Job drawing, mm, ordinate dimensions from the low corner. One solid piece. Coordinates: 2 decimals unless noted, no trailing zeros. Order: outer loops, then holes, each group sorted by start corner. A loop starts at its lowest first (then second) coordinate and runs counter-clockwise, first axis right, second up. Notation, with made-up numbers: M 55,4 L 114,4 A21 cw 114,43 Z; hole C 64,4.5 d6. An arc over 180 degrees is marked long. Write item = value, one per line. Start each with the question number.
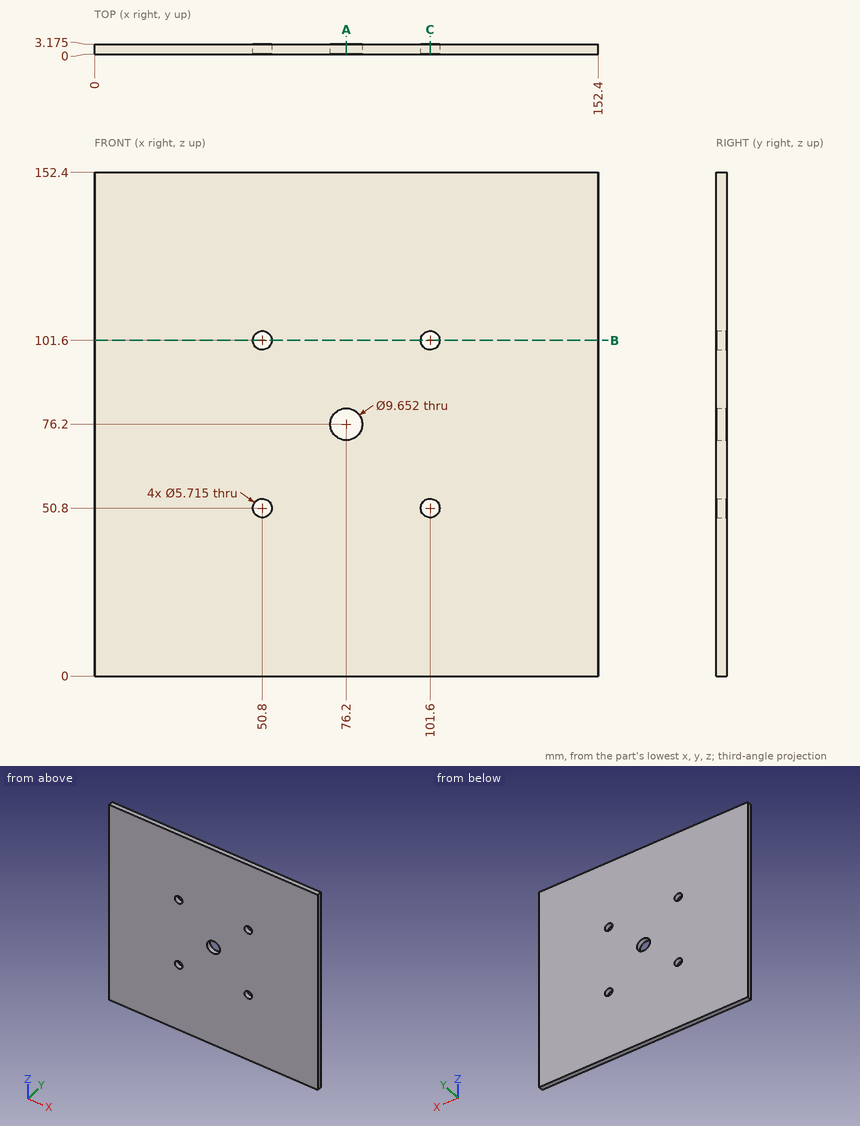
Item 1: Flat gauge pin, fed straight in: pin 1 (4.5 mm diameter, centred on x = 101.6, z = 101.6, fed in from -Y). Where does the tip first touch, or does it go through?
Item 2: Wall check: line 1 along Z through (x, y) = (101.6, 2.2); line 2 along X through (y, z) = (1.65, 100.5). Give the ranges that are in metal, low to high. Write a range as [from, to].
Item 3: Cut at A-A, the plane x = 76.2. Write the cut outline in (y, z) (3 decimals), and give its area (3 significant figures).
Item 4: Cut at B-B, the plane z = 101.6. Write the cut outline in (x, y) (1 decimal).
Item 5: Cut at C-C, the plane x = 101.6. Write the cut outline in (y, z) (1 decimal), and give its area (3 significant figures).
Filled sheet:
q1.pin_1 = through
q2.line_1 = [0, 47.94], [53.66, 98.74], [104.46, 152.4]
q2.line_2 = [0, 48.16], [53.44, 98.96], [104.24, 152.4]
q3.outline = M 0,0 L 3.175,0 L 3.175,71.374 L 0,71.374 Z; M 0,81.026 L 3.175,81.026 L 3.175,152.4 L 0,152.4 Z
q3.area = 453 mm2
q4.outline = M 0,0 L 47.9,0 L 47.9,3.2 L 0,3.2 Z; M 53.7,0 L 98.7,0 L 98.7,3.2 L 53.7,3.2 Z; M 104.5,0 L 152.4,0 L 152.4,3.2 L 104.5,3.2 Z
q5.outline = M 0,0 L 3.2,0 L 3.2,47.9 L 0,47.9 Z; M 0,53.7 L 3.2,53.7 L 3.2,98.7 L 0,98.7 Z; M 0,104.5 L 3.2,104.5 L 3.2,152.4 L 0,152.4 Z
q5.area = 448 mm2
